Input: part model. Units: mm. Frame: model coordinates. Give positions to 0.01 mm unless a question says otherwise; leave off trailing zeros. Loops run counter-clockwise (first coordinate to the right, second up) from the corner with the lowest first, then second, coordinate; pieces in that order, holes last.
from build123d import *

# Parameters (mm, degrees)
SKETCH1_W               = 203.2
SKETCH1_H               = 203.2
BOSS_EXTRUDE1_DEPTH     = 3.175
WHEEL_HOLES_REACH       = 5.175
SKETCH2_R               = 3.6
SKETCH2_R_2             = 2.625
BUILD_PLATE_HOLES_REACH = 5.175
SKETCH3_R               = 2.625
FILLET1_R               = 3.81
BELT_CLAMP_HOLES_REACH  = 5.175
SKETCH4_R               = 1.65


with BuildPart() as part:
    # Sketch1 → Boss-Extrude1 (new body)
    with BuildSketch(Plane(origin=(0, 0, 0), x_dir=(1, 0, 0), z_dir=(0, 1, 0))):
        with Locations((101.6, 101.6)):
            Rectangle(SKETCH1_W, SKETCH1_H)
    extrude(amount=BOSS_EXTRUDE1_DEPTH)

    # Sketch2 → wheel holes (cut, up to next)
    with BuildSketch(Plane(origin=(0, 3.175, 0), x_dir=(1, 0, 0), z_dir=(0, 1, 0)), mode=Mode.PRIVATE) as wheel_holes_sk1:
        with Locations((8.90143, 38.1)):
            Circle(SKETCH2_R)
    wheel_holes_tool1 = extrude(wheel_holes_sk1.sketch, amount=-WHEEL_HOLES_REACH, mode=Mode.PRIVATE) & part.part
    add(wheel_holes_tool1.solids().sort_by_distance((8.90143, 3.175, -38.1))[0], mode=Mode.SUBTRACT)
    # Sketch2 → wheel holes (cut, up to next)
    with BuildSketch(Plane(origin=(0, 3.175, 0), x_dir=(1, 0, 0), z_dir=(0, 1, 0)), mode=Mode.PRIVATE) as wheel_holes_sk2:
        with Locations((8.90143, 165.1)):
            Circle(SKETCH2_R)
    wheel_holes_tool2 = extrude(wheel_holes_sk2.sketch, amount=-WHEEL_HOLES_REACH, mode=Mode.PRIVATE) & part.part
    add(wheel_holes_tool2.solids().sort_by_distance((8.90143, 3.175, -165.1))[0], mode=Mode.SUBTRACT)
    # Sketch2 → wheel holes (cut, up to next)
    with BuildSketch(Plane(origin=(0, 3.175, 0), x_dir=(1, 0, 0), z_dir=(0, 1, 0)), mode=Mode.PRIVATE) as wheel_holes_sk3:
        with Locations((194.29857, 38.1)):
            Circle(SKETCH2_R_2)
    wheel_holes_tool3 = extrude(wheel_holes_sk3.sketch, amount=-WHEEL_HOLES_REACH, mode=Mode.PRIVATE) & part.part
    add(wheel_holes_tool3.solids().sort_by_distance((194.29857, 3.175, -38.1))[0], mode=Mode.SUBTRACT)
    # Sketch2 → wheel holes (cut, up to next)
    with BuildSketch(Plane(origin=(0, 3.175, 0), x_dir=(1, 0, 0), z_dir=(0, 1, 0)), mode=Mode.PRIVATE) as wheel_holes_sk4:
        with Locations((194.29857, 165.1)):
            Circle(SKETCH2_R_2)
    wheel_holes_tool4 = extrude(wheel_holes_sk4.sketch, amount=-WHEEL_HOLES_REACH, mode=Mode.PRIVATE) & part.part
    add(wheel_holes_tool4.solids().sort_by_distance((194.29857, 3.175, -165.1))[0], mode=Mode.SUBTRACT)

    # Sketch3 → build plate holes (cut, up to next)
    with BuildSketch(Plane.XZ, mode=Mode.PRIVATE) as build_plate_holes_sk1:
        with Locations((4.50088, -4.572)):
            Circle(SKETCH3_R)
    build_plate_holes_tool1 = extrude(build_plate_holes_sk1.sketch, amount=-BUILD_PLATE_HOLES_REACH, mode=Mode.PRIVATE) & part.part
    add(build_plate_holes_tool1.solids().sort_by_distance((4.50088, 0, -4.572))[0], mode=Mode.SUBTRACT)
    # Sketch3 → build plate holes (cut, up to next)
    with BuildSketch(Plane.XZ, mode=Mode.PRIVATE) as build_plate_holes_sk2:
        with Locations((4.50088, -198.628)):
            Circle(SKETCH3_R)
    build_plate_holes_tool2 = extrude(build_plate_holes_sk2.sketch, amount=-BUILD_PLATE_HOLES_REACH, mode=Mode.PRIVATE) & part.part
    add(build_plate_holes_tool2.solids().sort_by_distance((4.50088, 0, -198.628))[0], mode=Mode.SUBTRACT)
    # Sketch3 → build plate holes (cut, up to next)
    with BuildSketch(Plane.XZ, mode=Mode.PRIVATE) as build_plate_holes_sk3:
        with Locations((198.628, -101.6)):
            Circle(SKETCH3_R)
    build_plate_holes_tool3 = extrude(build_plate_holes_sk3.sketch, amount=-BUILD_PLATE_HOLES_REACH, mode=Mode.PRIVATE) & part.part
    add(build_plate_holes_tool3.solids().sort_by_distance((198.628, 0, -101.6))[0], mode=Mode.SUBTRACT)

    # Fillet1
    fillet1_edges = [part.edges().sort_by_distance(p)[0] for p in [
        (0, 1.5875, -203.2),
        (203.2, 1.5875, -203.2),
        (203.2, 1.5875, 0),
        (0, 1.5875, 0),
    ]]
    fillet(fillet1_edges, radius=FILLET1_R)

    # Sketch4 → belt clamp holes (cut, up to next)
    with BuildSketch(Plane(origin=(0, 3.175, 0), x_dir=(1, 0, 0), z_dir=(0, 1, 0)), mode=Mode.PRIVATE) as belt_clamp_holes_sk1:
        with Locations((94.6, 119.38)):
            Circle(SKETCH4_R)
    belt_clamp_holes_tool1 = extrude(belt_clamp_holes_sk1.sketch, amount=-BELT_CLAMP_HOLES_REACH, mode=Mode.PRIVATE) & part.part
    add(belt_clamp_holes_tool1.solids().sort_by_distance((94.6, 3.175, -119.38))[0], mode=Mode.SUBTRACT)
    # Sketch4 → belt clamp holes (cut, up to next)
    with BuildSketch(Plane(origin=(0, 3.175, 0), x_dir=(1, 0, 0), z_dir=(0, 1, 0)), mode=Mode.PRIVATE) as belt_clamp_holes_sk2:
        with Locations((108.6, 119.38)):
            Circle(SKETCH4_R)
    belt_clamp_holes_tool2 = extrude(belt_clamp_holes_sk2.sketch, amount=-BELT_CLAMP_HOLES_REACH, mode=Mode.PRIVATE) & part.part
    add(belt_clamp_holes_tool2.solids().sort_by_distance((108.6, 3.175, -119.38))[0], mode=Mode.SUBTRACT)
    # Sketch4 → belt clamp holes (cut, up to next)
    with BuildSketch(Plane(origin=(0, 3.175, 0), x_dir=(1, 0, 0), z_dir=(0, 1, 0)), mode=Mode.PRIVATE) as belt_clamp_holes_sk3:
        with Locations((108.6, 83.82)):
            Circle(SKETCH4_R)
    belt_clamp_holes_tool3 = extrude(belt_clamp_holes_sk3.sketch, amount=-BELT_CLAMP_HOLES_REACH, mode=Mode.PRIVATE) & part.part
    add(belt_clamp_holes_tool3.solids().sort_by_distance((108.6, 3.175, -83.82))[0], mode=Mode.SUBTRACT)
    # Sketch4 → belt clamp holes (cut, up to next)
    with BuildSketch(Plane(origin=(0, 3.175, 0), x_dir=(1, 0, 0), z_dir=(0, 1, 0)), mode=Mode.PRIVATE) as belt_clamp_holes_sk4:
        with Locations((94.6, 83.82)):
            Circle(SKETCH4_R)
    belt_clamp_holes_tool4 = extrude(belt_clamp_holes_sk4.sketch, amount=-BELT_CLAMP_HOLES_REACH, mode=Mode.PRIVATE) & part.part
    add(belt_clamp_holes_tool4.solids().sort_by_distance((94.6, 3.175, -83.82))[0], mode=Mode.SUBTRACT)


solid = part.part
(1) Ray query, probe 1 along X at (y, z) = (2.25, -119.38); probe 2 along X at (y, z) = (0.85, -38.1); probe 3 along Z at (x, y) = (110, 2.95). Return the intervals inside material, ascending.
Values follow:
probe 1: x = 0 to 92.95, 96.25 to 106.95, 110.25 to 203.2
probe 2: x = 0 to 5.3, 12.5 to 191.67, 196.92 to 203.2
probe 3: z = -203.2 to -120.25, -118.51 to -84.69, -82.95 to 0
(2) Mould query, pull axis Z, two halves, no side actions, for faces 1 (the flat face through (100, 0, -103)), 2 (the cylindrical face through (192.36, 1.61, -166.87)). Classes: +Z half, -Z half, draft (parallel to the pull), parting line (faces both ways), or undercut.
Values follow:
face 1: draft
face 2: undercut
(3) Cut plane B-B (z = -38.1). Return the cut outline in (x, y) (3 decimals).
Values follow:
outline: (0, 0) - (5.301, 0) - (5.301, 3.175) - (0, 3.175) - close; (12.501, 0) - (191.674, 0) - (191.674, 3.175) - (12.501, 3.175) - close; (196.924, 0) - (203.2, 0) - (203.2, 3.175) - (196.924, 3.175) - close
(4) Cut plane A-A (z = -101.6). Return the cut outline in (x, y) (3 decimals), and give its area (3 significant figures).
Values follow:
outline: (0, 0) - (196.003, 0) - (196.003, 3.175) - (0, 3.175) - close; (201.253, 0) - (203.2, 0) - (203.2, 3.175) - (201.253, 3.175) - close
area: 628 mm2
